Read the model definition and answer for the solid it produces. Units are mm, in the model's axes. A direction names the side the tool comes from. Give positions to 0.01 mm unless a question says otherwise; leave off trailing zeros. Order: outer loops, then holes, each group sorted by start corner. A loop starts at its lowest first (then second) coordinate and runs counter-clockwise, first axis right, second up. Notation, with made-up numbers: (25.25, -23) - (34.25, -23) arc R22 cw to (34.25, 5) - close; hole circle Ø6 at (-24, -17). An arc over 180 degrees is marked (long way). Write item = value, one per line.
```python
from build123d import *

# Parameters (mm, degrees)
EXTRUDE_1_DEPTH             = 15
SHELL_1_T                   = -1.5
SKETCH_3_R                  = 2.25
SKETCH_3_R_2                = 2.7
CUT_EXTRUDE_1_DEPTH         = 25
SKETCH_5_R                  = 2.25
SKETCH_5_R_2                = 2.7
CUT_EXTRUDE_3_DEPTH         = 20
HOLE_WIZARD_10_0_10_1_D     = 10
HOLE_WIZARD_10_0_10_1_DEPTH = 1.5
HOLE_WIZARD_10_0_10_2_D     = 10
HOLE_WIZARD_10_0_10_2_DEPTH = 1.5


with BuildPart() as part:
    # ｽｹｯﾁ1 → ﾎﾞｽ - 押し出し1 (new body)
    with BuildSketch(Plane.XY):
        Polygon((133.1152144, 365.731045751), (0, 0), (-14.095389312, 5.13030215), (119.019825089, 370.861347901), align=None)
    extrude(amount=EXTRUDE_1_DEPTH)

    # ｼｪﾙ1
    shell_1_openings = [part.faces().sort_by_distance(p)[0] for p in [
        (126.067519744, 368.296196826, 7.5),
        (-7.047694656, 2.565151075, 7.5),
    ]]
    offset(amount=SHELL_1_T, openings=shell_1_openings, kind=Kind.INTERSECTION)

    # ｽｹｯﾁ3 → ｶｯﾄ - 押し出し1 (cut)
    with BuildSketch(Plane.XY.offset(15)):
        with Locations((-4.482543581, 9.612845731)):
            Circle(SKETCH_3_R)
        with Locations((123.50236867, 361.24850217)):
            Circle(SKETCH_3_R)
        with Locations((113.24176437, 333.057723546)):
            Circle(SKETCH_3_R)
        with Locations((5.778060719, 37.803624354)):
            Circle(SKETCH_3_R)
        with Locations((12.618463585, 56.59747677)):
            Circle(SKETCH_3_R_2)
        with Locations((106.401361503, 314.263871131)):
            Circle(SKETCH_3_R_2)
    extrude(amount=-CUT_EXTRUDE_1_DEPTH, mode=Mode.SUBTRACT)

    # ｽｹｯﾁ5 → ｶｯﾄ - 押し出し3 (cut)
    with BuildSketch(Plane(origin=(-14.095389312, 5.13030215, 0), x_dir=(0, 0, 1), z_dir=(-0.939692621, 0.342020143, 0))):
        with Locations((7.5, 120.877716811)):
            Circle(SKETCH_5_R)
        with Locations((7.5, 90.877716811)):
            Circle(SKETCH_5_R)
        with Locations((7.5, 22.5)):
            Circle(SKETCH_5_R_2)
    extrude(amount=-CUT_EXTRUDE_3_DEPTH, mode=Mode.SUBTRACT)

    # Ø10.0 (10) 直径の穴1
    with Locations(Plane(origin=(0, 0, 0), x_dir=(0, 0, -1), z_dir=(0.939692621, -0.342020143, 0))):
        with Locations((-7.5, 22.5)):
            Hole(HOLE_WIZARD_10_0_10_1_D / 2, depth=HOLE_WIZARD_10_0_10_1_DEPTH)

    # Ø10.0 (10) 直径の穴2
    with Locations(Plane.XY.offset(15)):
        with Locations((106.401361503, 314.263871131), (12.618463585, 56.59747677)):
            Hole(HOLE_WIZARD_10_0_10_2_D / 2, depth=HOLE_WIZARD_10_0_10_2_DEPTH)


solid = part.part
```
1. Straight lines are drawn through the part: L1, parallel to X at y = 311.5, z = 9.25; L2, parallel to X at y = 181, z = 6.75; L3, parallel to X at y = 288, z = 0.5. For each, find the intervals that lie inside material, in ascending order. Write a range as [from, to].
Recorded:
L1 = [97.41, 99.01], [111.78, 113.38]
L2 = [49.92, 51.51], [64.28, 65.88]
L3 = [88.86, 104.82]
2. For faces 4 (the face through (60, 186, 13.5)), 5 (the face through (13.702, 51.716, 14.24)), 6 (the face through (60, 186, 0)), determine the directions among +Z, -Z, +X, -X, +Y, -Y from which every point of the face is accessible in a straight line to the end or side of a thin tool.
Recorded:
face_4 = none
face_5 = +Z
face_6 = -Z, +X, -X, +Y, -Y
3. Determine the mould class of faces 1 (the face through (60, 186, 15)), 2 (the face through (67.49, 185.43, 7.4)), 3 (the face through (5.311, 16.816, 6.416)) for opening direction Y: +Y half, -Y half, draft (parallel to the pull), parting line (faces both ways), or undercut.
Recorded:
face_1 = draft
face_2 = -Y half
face_3 = undercut
4. Section A-A (y = 282.5) is taken. Determine the outline of the cut face in (x, z).
Recorded:
outline = (86.86, 0) - (102.82, 0) - (102.82, 15) - (86.86, 15) - close; hole (88.46, 1.5) - (101.23, 1.5) - (101.23, 13.5) - (88.46, 13.5) - close
5. Flat-ended cylindrical pins translate along their axes: pin 1 (8 mm diameter, centred on y = 45.5, z = 13.5, fed in from +X); pin 2 (3 mm diameter, centred on y = 67.5, z = 8, fed in from +X); pin 3 (9 mm diameter, centred on x = 106.4, y = 314.26, fed in from +Z). Find the tip coordinate at first contact, or state that the pin passes through.
Recorded:
pin_1 = 18.02
pin_2 = 25.11
pin_3 = 1.5
6. Section B-B (x = 78.5) is taken. Determine the outline of the cut face in (y, z), and give its area (3 significant figures).
Recorded:
outline = (215.68, 0) - (259.53, 0) - (259.53, 15) - (215.68, 15) - close; hole (220.06, 1.5) - (255.15, 1.5) - (255.15, 13.5) - (220.06, 13.5) - close
area = 237 mm^2
